Geometry: final body of the model. Coordinates: model frame, mm. Coordinates: 2 decimals unless noted, no trailing zeros. Write each loop counter-clockwise with the first axis right and the second up, starting at its lowest first coordinate (ties: lowest second). Pieces come first, ordered by that corner, then holes. Notation, with made-up numbers: (-16.75, 64) -> (33.25, 64) arc R6 cw to (33.25, 75) -> close; hole circle Ø7 at (36.25, 5.25). An arc over 180 degrees is marked (long way). One line per item, written item: value.
Autodesk Inventor part; units mm, degrees
ref_plane "YZ Plane" through (0, 0, 0) normal (1, 0, 0) x (0, 1, 0)
ref_plane "XZ Plane" through (0, 0, 0) normal (0, 1, 0) x (-1, 0, 0)
ref_plane "XY Plane" through (0, 0, 0) normal (0, 0, 1) x (1, 0, 0)
sketch "Sketch1" plane through (0, 0, 0) normal (0, 0, 1) x (1, 0, 0)
  circle A0 centre (0, 0) radius 3.175
  dimension "d0" = 6.35
extrude "Extrusion1" add sketch "Sketch1" along normal blind 88.9
sketch "Sketch2" plane through (0, 0, 0) normal (0, 0, -1) x (-1, 0, 0)
  circle A0 centre (0, 0) radius 3.175
  circle A1 centre (0, 0) radius 4.7625
  dimension "d3" = 9.525
extrude "Extrusion2" add sketch "Sketch2" along normal blind 6.35 contours A0 | A1
sketch "Sketch3" plane through (0, 0, -6.35) normal (0, 0, -1) x (-1, 0, 0)
  circle A0 centre (0, 0) radius 4.7625
  line L0 (-1.3748, 2.3812) -> (1.3748, 2.3813)
  line L1 (1.3748, 2.3813) -> (2.7496, 0)
  line L2 (2.7496, 0) -> (1.3748, -2.3812)
  line L3 (1.3748, -2.3812) -> (-1.3748, -2.3812)
  line L4 (-1.3748, -2.3812) -> (-2.7496, 0)
  line L5 (-2.7496, 0) -> (-1.3748, 2.3812)
  dimension "d6" = 4.7625
extrude "Extrusion3" cut sketch "Sketch3" against normal blind 3.175 contours L0 L1 L2 L3 L4 L5
chamfer "Chamfer1" distance 0.508 angle 45 3 edges at (-3.175, 0, 88.9) (4.7625, 0, 0) (4.7625, 0, -6.35)
thread "Thread1"
properties part number "14-20 x750" material "Steel"
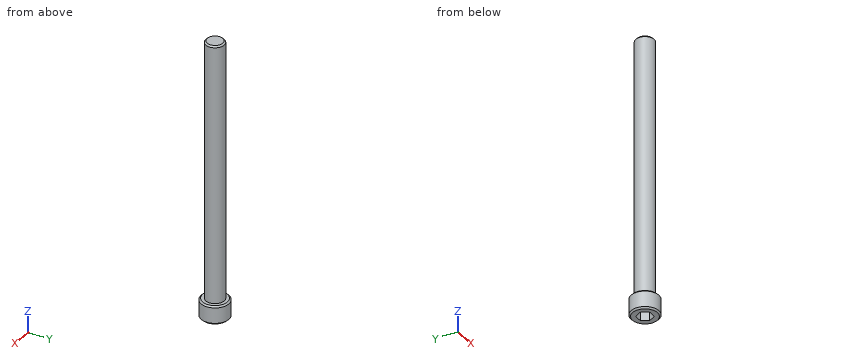
(1) Line query: line 1 (Z direction, x = 3.25, y = 2); line 2 (Z direction, x = 1.25, y = 0.25) (3 decimals); line 3 (Y direction, x = 0, z = 9) (3 decimals). Output: solid intervals per line, ascending. Write a range as [from, to].
Responses:
line 1: z = [-6.35, 0]
line 2: z = [-3.175, 88.9]
line 3: y = [-3.175, 3.175]
(2) First-contact query: pin 1 (1.5 mm diameter, centred on x = 3.5, z = 37, fed in from -Y); pin 2 (3 mm diameter, centred on x = -0.5, z = 70, fed in from -Y) (3 decimals); pin 3 (2 mm diameter, centred on y = -0.5, z = 67.5, fed in from -X) (3 decimals). Flat tips, straight axial feed; report the tip coordinate or a pass-through.
Responses:
pin 1: stops at y = -1.59
pin 2: stops at y = -3.175
pin 3: stops at x = -3.175
(3) Section A-A (z = 44). Return the cut outline in (x, y) (3 decimals), then the cut area to 3 significant figures.
Responses:
outline: circle Ø6.35 at (0, 0)
area: 31.7 mm2
